Could you check a few things on this drawing? It's one solid part, dimensions in mm from its lowest x, y, z. A direction names the side the tool comes from. Give positions to 0.01 mm unless a question says otherwise; leave off trailing zeros. Order: outer loops, then holes, each group sorted by start corner. A loop starts at its lowest first (then second) coordinate and runs counter-clockwise, first axis right, second up. Notation, with made-up numbers: (68.5, -4.75) -> (113.5, -4.75) arc R31 cw to (113.5, 19.25) -> close; hole circle Ø1 at (5, 57.5). An arc over 180 degrees is marked (long way). Write each question's results on one line, items separated by ' | '. Start each with the question number.
Q1. Imagine slicing it at C-C, the plane x = 8. Please give me the cut outline in (y, z).
Q2. For the marked faces 1 and 2, which set-ups out of +Z, -Z, +X, -X, +Y, -Y let a thin tool reach every point of the face, with its end or its side?
Q3. I need wall thicknesses on line 1 along Y through (x, z) = (1.75, 5); line 2 along Y through (x, z) = (2.5, 4); line 3 along X through (y, z) = (23, 12). Which ranges of each line are inside material? Lowest first, please. Write a range as [from, to].
Q4. Imagine slicing it at D-D, the plane z = 29.5. Please give me the cut outline in (x, y).
Q5. Imagine slicing it at A-A, the plane y = 23. Please give me the cut outline in (x, z), then the cut area to 3 significant figures.
Q6. Imagine slicing it at B-B, the plane z = 5. Please give me the cut outline in (x, y).
Q7. I'm going to push flat-ended pins straight in: pin 1 (7.5 mm diameter, centred on y = 16.5, z = 17, fed in from +X); pin 2 (4 mm diameter, centred on x = 17.45, z = 24.05, fed in from +Y); pin 3 (3 mm diameter, centred on y = 10, z = 27, fed in from -X). Where does each tip first touch, or does it pass through?
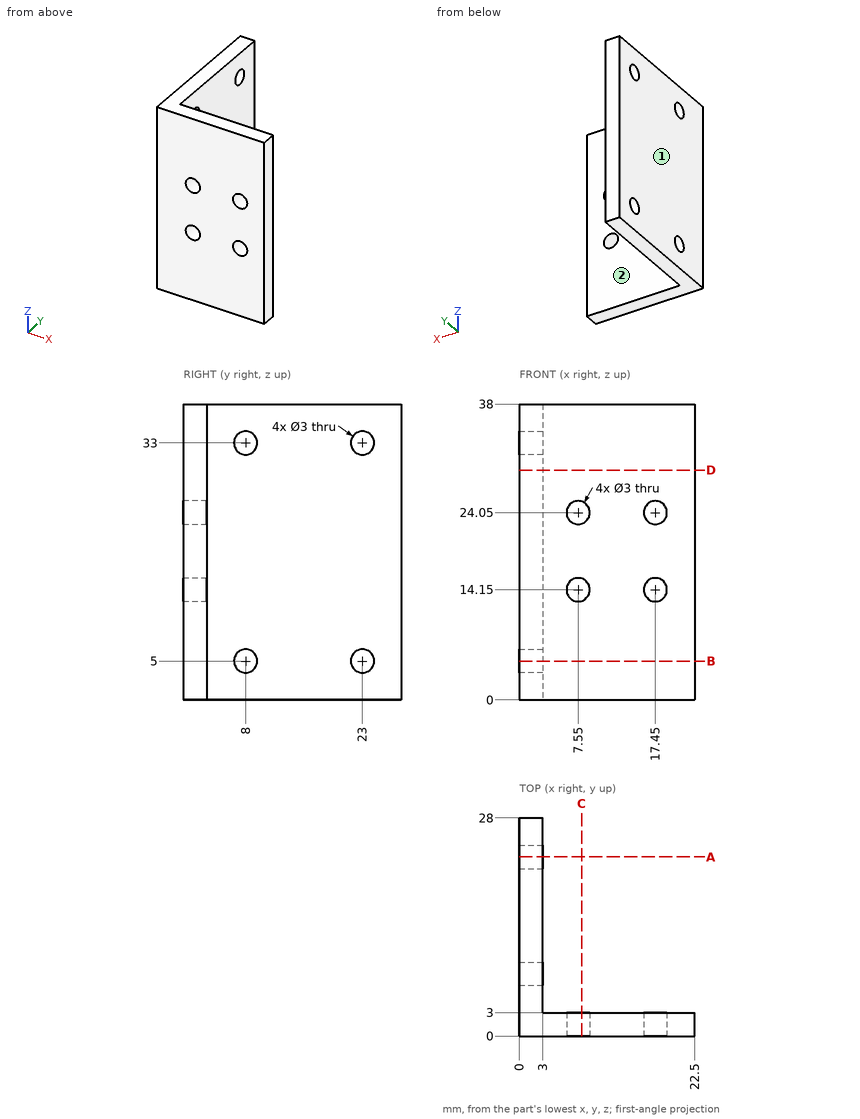
Geometry check:
1) outline: (0, 0) -> (3, 0) -> (3, 12.72) -> (0, 12.72) -> close; (0, 15.58) -> (3, 15.58) -> (3, 22.62) -> (0, 22.62) -> close; (0, 25.48) -> (3, 25.48) -> (3, 38) -> (0, 38) -> close
2) face 1: +Z, -Z, -X, +Y, -Y | face 2: +Z, -Z, +X, +Y
3) line 1: [0, 6.5], [9.5, 21.5], [24.5, 28] | line 2: [0, 6.88], [9.12, 21.88], [24.12, 28] | line 3: [0, 3]
4) outline: (0, 0) -> (22.5, 0) -> (22.5, 3) -> (3, 3) -> (3, 28) -> (0, 28) -> close
5) outline: (0, 0) -> (3, 0) -> (3, 3.5) -> (0, 3.5) -> close; (0, 6.5) -> (3, 6.5) -> (3, 31.5) -> (0, 31.5) -> close; (0, 34.5) -> (3, 34.5) -> (3, 38) -> (0, 38) -> close | area: 96.0 mm²
6) outline: (0, 0) -> (22.5, 0) -> (22.5, 3) -> (3, 3) -> (3, 6.5) -> (0, 6.5) -> close; (0, 9.5) -> (3, 9.5) -> (3, 21.5) -> (0, 21.5) -> close; (0, 24.5) -> (3, 24.5) -> (3, 28) -> (0, 28) -> close
7) pin 1: x = 3 | pin 2: y = 3 | pin 3: x = 0
